```python
from build123d import *

# Parameters (mm, degrees)
BOSS_EXTRUDE1_DEPTH = 25.4
SHELL3_T            = -2


with BuildPart() as part:
    # Sketch1 → Boss-Extrude1 (new body)
    with BuildSketch(Plane(origin=(0, 0, 0), x_dir=(1, 0, 0), z_dir=(0, 1, 0))):
        Polygon((-90.556063278, -9.208067905), (-72.595551035, 21.900451829), (141.48342448, 21.900451829), (159.443936722, -9.208067905), align=None)
    extrude(amount=BOSS_EXTRUDE1_DEPTH)

    # Shell3
    shell3_openings = [part.faces().sort_by_distance(p)[0] for p in [
        (150.463680601, 12.7, -6.346191962),
    ]]
    offset(amount=SHELL3_T, openings=shell3_openings, kind=Kind.INTERSECTION)


solid = part.part
```
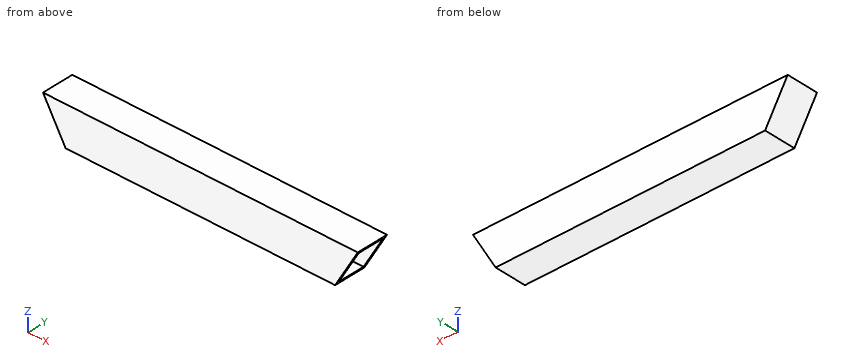
Design review of the part built by this model. Coordinates are the model's own, in mm. Give positions to 0.01 mm unless a question says otherwise; leave off trailing zeros. Order: outer loops, then holes, each group sorted by start corner. A loop starts at its lowest first (then second) coordinate and runs counter-clockwise, first axis right, second up. Notation, with made-up numbers: (-30.5, -5.75) - (-24.5, -5.75) arc R20 cw to (-24.5, 2.25) - close; hole circle Ø7 at (71.5, -36.5). An arc over 180 degrees is marked (long way). Use a Markdown table: item, result. Add a question column.
(1) Clearance check with flat-ended pins moving along their axes: P1, Ø12, axis at y = 5, z = -10.5, coming from the -X side; P2, Ø5, axis at y = 18.5, z = -14.5, coming from the +X side; P3, Ø2, axis at y = 21, z = 3, coming from the +X side. State where each tip first meets the part, or that it passes through.
(2) Add section C-C on z = -8. Give the boundary of the cut face in (x, y), then the cut area to 3 significant figures.
(3) Add section D-D on x = -75. Give the boundary of the cut face in (y, z), then the cut area to 3 significant figures.
(4) Add section A-A on y = 10.5. Give the boundary of the cut face in (x, z).
(5) Add section B-B on x = 137. Give the boundary of the cut face in (y, z), then the cut area to 3 significant figures.
(6) Wall thickness on probe 1 along Z at (x, y) = (110.5, 12.25); probe 2 along Y at (x, z) = (-10, -1.5); probe 3 along Z at (x, y) = (-79.5, 4): over which ranges is each line inside the solid? List them lowest first. Write a range as [from, to].
Report:
| question | item | result |
|---|---|---|
| 1 | P1 | stops at x = -82.64 |
| 1 | P2 | stops at x = -73.12 |
| 1 | P3 | stops at x = -84.09 |
| 2 | outline | (-80.62, 0) - (149.51, 0) - (149.51, 2) - (-78.31, 2) - (-78.31, 23.4) - (149.51, 23.4) - (149.51, 25.4) - (-80.62, 25.4) - close |
| 2 | area | 970 mm² |
| 3 | outline | (0, -17.74) - (25.4, -17.74) - (25.4, 9.21) - (0, 9.21) - close; hole (2, -13.74) - (23.4, -13.74) - (23.4, 7.21) - (2, 7.21) - close |
| 3 | area | 236 mm² |
| 4 | outline | (-90.56, 9.21) - (-72.6, -21.9) - (141.48, -21.9) - (142.64, -19.9) - (-71.44, -19.9) - (-87.09, 7.21) - (158.29, 7.21) - (159.44, 9.21) - close |
| 5 | outline | (0, -21.9) - (25.4, -21.9) - (25.4, 9.21) - (0, 9.21) - close; hole (2, -19.9) - (23.4, -19.9) - (23.4, 7.21) - (2, 7.21) - close |
| 5 | area | 210 mm² |
| 6 | probe 1 | z = [-21.9, -19.9], [7.21, 9.21] |
| 6 | probe 2 | y = [0, 2], [23.4, 25.4] |
| 6 | probe 3 | z = [-9.94, -5.94], [7.21, 9.21] |
